from build123d import *

# Parameters (mm, degrees)
IZIM1_R                          = 0.25
Y_KSEKLIK_EKSTR_ZYON1_DEPTH      = 2.5
IZIM2_R                          = 0.25
Y_KSEKLIK_EKSTR_ZYON2_DEPTH      = 5.5
Y_KSEKLIK_EKSTR_ZYON2_DEPTH_BACK = 5


with BuildPart() as part:
    # Çizim1 → Yükseklik-Ekstrüzyon1 (new body)
    with BuildSketch(Plane(origin=(0, 0, 0), x_dir=(1, 0, 0), z_dir=(0, 1, 0))):
        with BuildLine():
            Line((-7.3, 1.25), (-5.1, 1.25))
            ThreePointArc((-5.1, 1.25), (-5, 1.15), (-4.9, 1.25))
            Line((-4.9, 1.25), (-2.6, 1.25))
            ThreePointArc((-2.6, 1.25), (-2.5, 1.15), (-2.4, 1.25))
            Line((-2.4, 1.25), (-0.1, 1.25))
            ThreePointArc((-0.1, 1.25), (0, 1.15), (0.1, 1.25))
            Line((0.1, 1.25), (2.4, 1.25))
            ThreePointArc((2.4, 1.25), (2.5, 1.15), (2.6, 1.25))
            Line((2.6, 1.25), (4.9, 1.25))
            ThreePointArc((4.9, 1.25), (5, 1.15), (5.1, 1.25))
            Line((5.1, 1.25), (7.3, 1.25))
            ThreePointArc((7.3, 1.25), (7.441421356, 1.191421356), (7.5, 1.05))
            Line((7.5, 1.05), (7.5, -1.05))
            ThreePointArc((7.5, -1.05), (7.441421356, -1.191421356), (7.3, -1.25))
            Line((7.3, -1.25), (5.1, -1.25))
            ThreePointArc((5.1, -1.25), (5, -1.15), (4.9, -1.25))
            Line((4.9, -1.25), (2.6, -1.25))
            ThreePointArc((2.6, -1.25), (2.5, -1.15), (2.4, -1.25))
            Line((2.4, -1.25), (0.1, -1.25))
            ThreePointArc((0.1, -1.25), (0, -1.15), (-0.1, -1.25))
            Line((-0.1, -1.25), (-2.4, -1.25))
            ThreePointArc((-2.4, -1.25), (-2.5, -1.15), (-2.6, -1.25))
            Line((-2.6, -1.25), (-4.9, -1.25))
            ThreePointArc((-4.9, -1.25), (-5, -1.15), (-5.1, -1.25))
            Line((-5.1, -1.25), (-7.3, -1.25))
            ThreePointArc((-7.3, -1.25), (-7.441421356, -1.191421356), (-7.5, -1.05))
            Line((-7.5, -1.05), (-7.5, 1.05))
            ThreePointArc((-7.5, 1.05), (-7.441421356, 1.191421356), (-7.3, 1.25))
        make_face()
        with Locations((-1.25, 0)):
            Circle(IZIM1_R, mode=Mode.SUBTRACT)
        with Locations((-3.75, 0)):
            Circle(IZIM1_R, mode=Mode.SUBTRACT)
        with Locations((-6.25, 0)):
            Circle(IZIM1_R, mode=Mode.SUBTRACT)
        with Locations((6.25, 0)):
            Circle(IZIM1_R, mode=Mode.SUBTRACT)
        with Locations((3.75, 0)):
            Circle(IZIM1_R, mode=Mode.SUBTRACT)
        with Locations((1.25, 0)):
            Circle(IZIM1_R, mode=Mode.SUBTRACT)
    extrude(amount=Y_KSEKLIK_EKSTR_ZYON1_DEPTH)

    # Çizim2 → Yükseklik-Ekstrüzyon2 (add, two sides)
    with BuildSketch(Plane(origin=(0, 2.5, 0), x_dir=(1, 0, 0), z_dir=(0, 1, 0))) as y_kseklik_ekstr_zyon2_sk:
        with Locations((-6.25, 0)):
            Circle(IZIM2_R)
        with Locations((-3.75, 0)):
            Circle(IZIM2_R)
        with Locations((-1.25, 0)):
            Circle(IZIM2_R)
        with Locations((1.25, 0)):
            Circle(IZIM2_R)
        with Locations((3.75, 0)):
            Circle(IZIM2_R)
        with Locations((6.25, 0)):
            Circle(IZIM2_R)
    extrude(amount=Y_KSEKLIK_EKSTR_ZYON2_DEPTH)
    extrude(y_kseklik_ekstr_zyon2_sk.sketch, amount=-Y_KSEKLIK_EKSTR_ZYON2_DEPTH_BACK)


solid = part.part
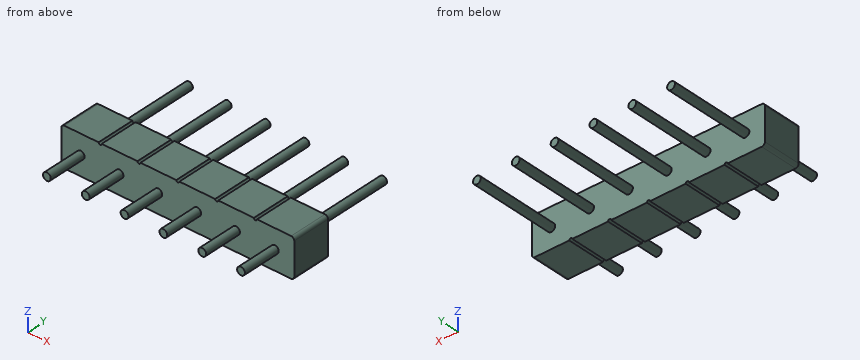
The listing builds one solid part. Answer for the finished solid, in the listing's coordinates (mm). Coordinates: 2 decimals unless noted, no trailing zeros. Loops run counter-clockwise (first coordinate to the right, second up) from the corner with the lowest first, then second, coordinate; pieces in that order, holes last.
1) Find section C-C on z = -0.75. Write down the section's boundary in (x, y).
2) Find section B-B on x = -6.25. Write down the section's boundary in (y, z), then the cut area to 4 significant figures.
3) Find section A-A on y = -1.75. Write down the section's boundary in (x, z), then the cut area to 3 significant figures.
4) Flat-ended cylindrical pins translate along their axes: pin 1 Ø1.5 at (y, z) = (6.5, -0.5) entering from +X; pin 2 Ø2 at (x, y) = (3.5, 6) entering from -Z. Find the tip coordinate at first contact, or state that the pin passes through.
5) Find the intervals of material crossed by L1, parallel to X at y = -1.25, z = 0.2; L2, parallel to Y at x = 2.5, z = 0.6, in increasing order.
6) Find section D-D on x = -4.75. Write down the section's boundary in (y, z).
Values:
1. outline: (-7.5, 0) - (7.5, 0) - (7.5, 2.5) - (-7.5, 2.5) - close
2. outline: (-2.5, -0.25) - (0, -0.25) - (0, -1.25) - (2.5, -1.25) - (2.5, -0.25) - (8, -0.25) - (8, 0.25) - (2.5, 0.25) - (2.5, 1.25) - (0, 1.25) - (0, 0.25) - (-2.5, 0.25) - close
2. area: 10.25 mm2
3. outline: circle Ø0.5 at (-6.25, 0); circle Ø0.5 at (-3.75, 0); circle Ø0.5 at (-1.25, 0); circle Ø0.5 at (1.25, 0); circle Ø0.5 at (3.75, 0); circle Ø0.5 at (6.25, 0)
3. area: 1.18 mm2
4. pin 1: stops at x = 6.5
4. pin 2: stops at z = -0.25
5. L1: x = -6.4 to -6.1, -3.9 to -3.6, -1.4 to -1.1, 1.1 to 1.4, 3.6 to 3.9, 6.1 to 6.4
5. L2: y = 0 to 2.5
6. outline: (0, -1.25) - (2.5, -1.25) - (2.5, 1.25) - (0, 1.25) - close
